Could you check a few things on this model? Use its own coordinates, in mm. Coordinates: 2 decimals unless noted, no trailing zeros. Loops run counter-clockwise (first coordinate to the right, second up) from the corner with the lowest first, then second, coordinate; pieces in that order, holes last. Notation, with made-up numbers: M -17.75,-15.75 L 36.25,-15.75 A21 cw 36.25,4.25 Z; hole C 37,-20.75 d11. An arc over 180 degrees is marked long. Use one line per item in the form item = value. Start each with the question number.
```python
from build123d import *

# Parameters (mm, degrees)
SKETCH_1_W          = 168
SKETCH_1_H          = 167
EXTRUDE_1_DEPTH     = 2
SKETCH_2_R          = 2.2
CUT_EXTRUDE_1_DEPTH = 2
SKETCH_3_W          = 168
SKETCH_3_H          = 2
CUT_EXTRUDE_2_DEPTH = 2
SKETCH_4_R          = 2.2
CUT_EXTRUDE_3_DEPTH = 2
SKETCH_6_R          = 2.2
CUT_EXTRUDE_5_DEPTH = 10
SKETCH_7_R          = 2.2
CUT_EXTRUDE_6_DEPTH = 10


with BuildPart() as part:
    # ｽｹｯﾁ1 → ﾎﾞｽ - 押し出し1 (new body)
    with BuildSketch(Plane.XY):
        Rectangle(SKETCH_1_W, SKETCH_1_H)
    extrude(amount=EXTRUDE_1_DEPTH)

    # ｽｹｯﾁ2 → ｶｯﾄ - 押し出し1 (cut)
    with BuildSketch(Plane.XY.offset(2)):
        with Locations((76, -68.5)):
            Circle(SKETCH_2_R)
        with Locations((76, -8.5)):
            Circle(SKETCH_2_R)
        with Locations((76, 51.5)):
            Circle(SKETCH_2_R)
    extrude(amount=-CUT_EXTRUDE_1_DEPTH, mode=Mode.SUBTRACT)

    # ｽｹｯﾁ3 → ｶｯﾄ - 押し出し2 (cut)
    with BuildSketch(Plane(origin=(0, 83.5, 0), x_dir=(1, 0, 0), z_dir=(0, 1, 0))):
        with Locations((0, -1)):
            Rectangle(SKETCH_3_W, SKETCH_3_H)
    extrude(amount=-CUT_EXTRUDE_2_DEPTH, mode=Mode.SUBTRACT)

    # ｽｹｯﾁ4 → ｶｯﾄ - 押し出し3 (cut)
    with BuildSketch(Plane.XY.offset(2)):
        with BuildLine():
            ThreePointArc((-6.8, -76), (-9, -73.8), (-11.2, -76))
            Line((-11.2, -76), (-9, -76))
            Line((-9, -76), (-6.8, -76))
        make_face()
        with BuildLine():
            Line((-9, -76), (-11.2, -76))
            ThreePointArc((-11.2, -76), (-9, -78.2), (-6.8, -76))
            Line((-6.8, -76), (-9, -76))
        make_face()
        with BuildLine():
            ThreePointArc((-66.8, -76), (-69, -73.8), (-71.2, -76))
            Line((-71.2, -76), (-69, -76))
            Line((-69, -76), (-66.8, -76))
        make_face()
        with BuildLine():
            Line((-69, -76), (-71.2, -76))
            ThreePointArc((-71.2, -76), (-69, -78.2), (-66.8, -76))
            Line((-66.8, -76), (-69, -76))
        make_face()
        with Locations((51, -76)):
            Circle(SKETCH_4_R)
    extrude(amount=-CUT_EXTRUDE_3_DEPTH, mode=Mode.SUBTRACT)

    # ｽｹｯﾁ6 → ｶｯﾄ - 押し出し5 (cut)
    with BuildSketch(Plane(origin=(0, 0, 0), x_dir=(-1, 0, 0), z_dir=(0, 0, -1))):
        with Locations((74, 52.5)):
            Circle(SKETCH_6_R)
    extrude(amount=-CUT_EXTRUDE_5_DEPTH, mode=Mode.SUBTRACT)

    # ｽｹｯﾁ7 → ｶｯﾄ - 押し出し6 (cut)
    with BuildSketch(Plane(origin=(0, 0, 0), x_dir=(-1, 0, 0), z_dir=(0, 0, -1))):
        with Locations((74, -53.5)):
            Circle(SKETCH_7_R)
    extrude(amount=-CUT_EXTRUDE_6_DEPTH, mode=Mode.SUBTRACT)


solid = part.part
```
Item 1: Please list where these lines run through material, in increasing order: line 1 along Y through (x, z) = (76, 1.65); line 2 along Y through (x, z) = (-69, 1.45); line 3 along X through (y, z) = (-7.5, 1.2).
Item 2: I want a section at A-A (y = -76). Write out the boundary of the cut face in (x, z).
Item 3: I'm going to push a flat-ended pin straight in: P1, Ø2.5, axis at x = -74, y = -53.5, coming from the +Z side. Where does the tip first touch, or does it pass through?
Item 4: Thinking about a two-plate mould opening in Y: for faces 1 (the flat face through (-1, 0, 0)), 2 (the cylindrical face through (78.1, -7.84, 1.01)), which applies, pulls with the +Y half, pulls with the -Y half, needs draft (parallel to the pull), parting line crosses it, or undercut?
Item 5: I want a section at C-C (x = -74). Write out the boundary of the cut face in (y, z).
Item 6: I want a section at B-B (x = 76). Write out the boundary of the cut face in (y, z).
Worked answers:
q1.line_1 = -83.5 to -70.7, -66.3 to -10.7, -6.3 to 49.3, 53.7 to 81.5
q1.line_2 = -83.5 to -78.2, -73.8 to 81.5
q1.line_3 = -84 to 74.04, 77.96 to 84
q2.outline = M -84,0 L -71.2,0 L -71.2,2 L -84,2 Z; M -66.8,0 L -11.2,0 L -11.2,2 L -66.8,2 Z; M -6.8,0 L 48.8,0 L 48.8,2 L -6.8,2 Z; M 53.2,0 L 84,0 L 84,2 L 53.2,2 Z
q3.P1 = through
q4.face_1 = needs draft
q4.face_2 = undercut
q5.outline = M -83.5,0 L -55.7,0 L -55.7,2 L -83.5,2 Z; M -51.3,0 L 50.3,0 L 50.3,2 L -51.3,2 Z; M 54.7,0 L 81.5,0 L 81.5,2 L 54.7,2 Z
q6.outline = M -83.5,0 L -70.7,0 L -70.7,2 L -83.5,2 Z; M -66.3,0 L -10.7,0 L -10.7,2 L -66.3,2 Z; M -6.3,0 L 49.3,0 L 49.3,2 L -6.3,2 Z; M 53.7,0 L 81.5,0 L 81.5,2 L 53.7,2 Z
